Check sheet for the modelled part. Datum: model origin and axes. Units: mm. Face numbers are marked on the shaded views. A direction names the side the tool comes from. Round coordinates to 2 decimals unless told otherwise and drop trailing zeros. Loops run counter-clockwise (first coordinate to the right, second up) from the corner with the lowest first, then second, coordinate; pieces in that order, holes last. Notation, with made-up numbers: (-19.75, -23.5) -> (5.25, -23.5) arc R20 cw to (5.25, -13.5) -> close; hole circle Ø6 at (13.5, 89). An arc over 180 degrees is marked (long way). Use one line per item in the form item = value. Start each with the question number.
(1) Material ranges on probe 1 along Z at (x, y) = (29.95, 8); probe 2 along Y at (x, z) = (14, 1.3); probe 3 along Y at (x, z) = (8, 0.8), recorded low to high. Write a range as [from, to].
(2) Sectioned sample at C-C (z = 19.5). Record the cut outline in (x, y), and give its area (3 significant figures).
(3) Go/stop test with flat-tipped pins: pin 1 (1.8 mm diameter, centred on y = 8, z = 25.5, fed in from +X); pin 2 (4 mm diameter, centred on x = 22.5, y = 5, fed in from +Z); pin 3 (1.2 mm diameter, centred on x = 1, z = 5.5, fed in from -Y). Record where each tip stops, or that it passes through.
(4) Sectioned sample at A-A (x = 14). Record the cut outline in (y, z), and give its area (3 significant figures).
(5) Sectioned sample at D-D (z = 11.75). Record the cut outline in (x, y), and give its area (3 significant figures).
(6) Draft check along Z on the marked faces 6, 7 and 8. Enter one of: released by +Z, released by -Z, zero draft, split by the parting line, or undercut.
(7) Set-up check for the marked faces 1, 2, 3, 4 and 5: record each of +Z, -Z, +X, -X, +Y, -Y from which the full face is reachable in a straight line by a thin tool's end or side.
(8) Sectioned sample at B-B (y = 8). Record the cut outline in (x, z).
from build123d import *

# Parameters (mm, degrees)
SKETCH_W        = 31
SKETCH_H        = 16
SKETCH_R        = 1
PAD_DEPTH       = 2.5
SKETCH001_W     = 2.5
SKETCH001_H     = 16
PAD001_DEPTH    = 25
SKETCH002_R     = 1
POCKET_DEPTH    = 5
SKETCH003_W     = 2.5
SKETCH003_H     = 16
PAD002_DEPTH    = 25
POCKET001_DEPTH = 5
SKETCH005_R     = 3.25
PAD003_DEPTH    = 2


with BuildPart() as part:
    # Sketch → Pad (new body)
    with BuildSketch(Plane.XY):
        with Locations((15.5, 8)):
            Rectangle(SKETCH_W, SKETCH_H)
        with Locations((14, 14)):
            Circle(SKETCH_R, mode=Mode.SUBTRACT)
        with Locations((8, 8)):
            Circle(SKETCH_R, mode=Mode.SUBTRACT)
        with Locations((14, 2)):
            Circle(SKETCH_R, mode=Mode.SUBTRACT)
        with Locations((20, 8)):
            Circle(SKETCH_R, mode=Mode.SUBTRACT)
    extrude(amount=PAD_DEPTH)

    # Sketch001 (on Face10 of Pad) → Pad001 (join)
    with BuildSketch(Plane.XY.offset(2.5)):
        with Locations((29.75, 8)):
            Rectangle(SKETCH001_W, SKETCH001_H)
    extrude(amount=PAD001_DEPTH)

    # Sketch002 (on Face8 of Pad001) → Pocket (cut)
    with BuildSketch(Plane.YZ.offset(31)):
        with Locations((8, 25.5)):
            Circle(SKETCH002_R)
        with Locations((2, 19.5)):
            Circle(SKETCH002_R)
        with Locations((14, 19.5)):
            Circle(SKETCH002_R)
        with Locations((8, 13.5)):
            Circle(SKETCH002_R)
        with BuildLine():
            ThreePointArc((4, 27.5), (1.171573, 26.328427), (0, 23.5))
            Line((0, 23.5), (-2, 23.5))
            Line((-2, 23.5), (-2, 29.5))
            Line((-2, 29.5), (4, 29.5))
            Line((4, 29.5), (4, 27.5))
        make_face()
        with BuildLine():
            ThreePointArc((16, 23.5), (14.828427, 26.328427), (12, 27.5))
            Line((12, 29.5), (12, 27.5))
            Line((18, 29.5), (12, 29.5))
            Line((18, 23.5), (18, 29.5))
            Line((16, 23.5), (18, 23.5))
        make_face()
    extrude(amount=-POCKET_DEPTH, mode=Mode.SUBTRACT)

    # Sketch003 (on Face5 of Pocket) → Pad002 (join)
    with BuildSketch(Plane.XY.offset(2.5)):
        with Locations((1.25, 8)):
            Rectangle(SKETCH003_W, SKETCH003_H)
    extrude(amount=PAD002_DEPTH)

    # Sketch004 (on Face9 of Pad002) → Pocket001 (cut)
    with BuildSketch(Plane(origin=(0, 0, 0), x_dir=(0, -1, 0), z_dir=(-1, 0, 0))):
        with BuildLine():
            ThreePointArc((-2, 14.208497), (-8, 27.5), (-14, 14.208497))
            Line((-14, 14.208497), (-14, 2.5))
            Line((-14, 2.5), (-18, 2.5))
            Line((-18, 2.5), (-18, 29.5))
            Line((-18, 29.5), (2, 29.5))
            Line((2, 29.5), (2, 2.5))
            Line((-2, 2.5), (2, 2.5))
            Line((-2, 14.208497), (-2, 2.5))
        make_face()
    extrude(amount=-POCKET001_DEPTH, mode=Mode.SUBTRACT)

    # Sketch005 (on Face19 of Pocket001) → Pad003 (join)
    with BuildSketch(Plane.YZ.offset(2.5)):
        with Locations((8, 19.5)):
            Circle(SKETCH005_R)
    extrude(amount=PAD003_DEPTH)


solid = part.part
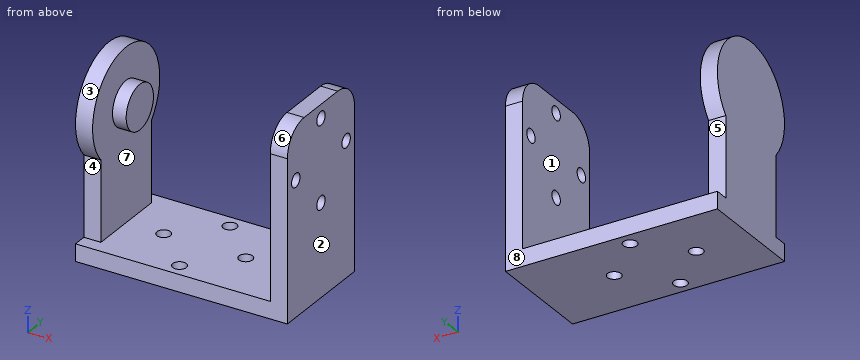
Checks:
q1.probe_1 = [0, 12.5], [14.5, 24.5], [26.5, 27.5]
q1.probe_2 = [0, 1], [3, 13], [15, 16]
q1.probe_3 = [0, 7], [9, 16]
q2.outline = (0, 0) -> (2.5, 0) -> (2.5, 4.75) -> (4.5, 4.75) -> (4.5, 11.25) -> (2.5, 11.25) -> (2.5, 16) -> (0, 16) -> close; (28.5, 0) -> (31, 0) -> (31, 1) -> (28.5, 1) -> close; (28.5, 3) -> (31, 3) -> (31, 13) -> (28.5, 13) -> close; (28.5, 15) -> (31, 15) -> (31, 16) -> (28.5, 16) -> close
q2.area = 83.0 mm2
q3.pin_1 = 2.5
q3.pin_2 = 2.5
q3.pin_3 = 2
q4.outline = (0, 0) -> (1, 0) -> (1, 2.5) -> (0, 2.5) -> close; (3, 0) -> (13, 0) -> (13, 2.5) -> (3, 2.5) -> close; (15, 0) -> (16, 0) -> (16, 2.5) -> (15, 2.5) -> close
q4.area = 30.0 mm2
q5.outline = (0, 2) -> (2.5, 2) -> (2.5, 14) -> (0, 14) -> close; (28.5, 0) -> (31, 0) -> (31, 16) -> (28.5, 16) -> close
q5.area = 70.0 mm2
q6.face_6 = released by +Z
q6.face_7 = undercut
q6.face_8 = zero draft
q7.face_1 = +Z, +Y, -Y
q7.face_2 = +Z, -Z, +X, +Y, -Y
q7.face_3 = -X
q7.face_4 = -X, -Y
q7.face_5 = -X, +Y
q8.outline = (0, 0) -> (7, 0) -> (7, 2.5) -> (2.5, 2.5) -> (2.5, 16.25) -> (4.5, 16.25) -> (4.5, 22.75) -> (2.5, 22.75) -> (2.5, 27.5) -> (0, 27.5) -> close; (9, 0) -> (19, 0) -> (19, 2.5) -> (9, 2.5) -> close; (21, 0) -> (31, 0) -> (31, 12.5) -> (28.5, 12.5) -> (28.5, 2.5) -> (21, 2.5) -> close; (28.5, 14.5) -> (31, 14.5) -> (31, 24.5) -> (28.5, 24.5) -> close; (28.5, 26.5) -> (31, 26.5) -> (31, 27.5) -> (28.5, 27.5) -> close
